Part model, mm, in its own coordinate system. A direction names the side the tool comes from. Give positions to 0.01 mm unless a question says otherwise; leave off trailing zeros. Order: outer loops, then holes, each group sorted by start corner. A loop starts at its lowest first (then second) coordinate and runs counter-clockwise, first axis right, second up. Notation, with made-up numbers: M 64.5,-13.5 L 111.5,-13.5 A25 cw 111.5,7.5 Z; hole C 21.25,51 d7. An arc over 180 degrees is marked long. One line per question, with ' | ' between items.
```python
from build123d import *

# Parameters (mm, degrees)
F0_R     = 11.4935
F0_R_2   = 9.017
F1_DEPTH = 4.064
F2_R     = 13.9954
F2_R_2   = 9.0043
F3_DEPTH = 69.85
F4_R     = 11.6713
F5_DEPTH = 7.62
F6_R     = 1.143
F7_DEPTH = 13.9964


with BuildPart() as f1:
    # F0 (on Top) → F1 (new body)
    with BuildSketch(Plane.XY):
        Circle(F0_R)
        Circle(F0_R_2, mode=Mode.SUBTRACT)
    extrude(amount=F1_DEPTH)

    # F2 (on face) → F3 (join)
    with BuildSketch(Plane(origin=(0, 0, 0), x_dir=(1, 0, 0), z_dir=(0, 0, -1))):
        Circle(F2_R)
        Circle(F2_R_2, mode=Mode.SUBTRACT)
    extrude(amount=F3_DEPTH)

    # F4 (on face) → F5 (cut)
    with BuildSketch(Plane(origin=(0, 0, -69.85), x_dir=(1, 0, 0), z_dir=(0, 0, -1))):
        Circle(F4_R)
    extrude(amount=-F5_DEPTH, mode=Mode.SUBTRACT)

    # F6 (on Right) → F7 (cut, through all)
    with BuildSketch(Plane.YZ):
        with Locations((0, -67.31)):
            Circle(F6_R)
    extrude(amount=F7_DEPTH, mode=Mode.SUBTRACT)


solid = f1.part
```
1. Slice it at D-D on z = -41. Give the cut face in (x, y).
Worked out:
outline: C 0,0 d27.99; hole C 0,0 d18.01
2. Tool access for faces 5 (the flat face through (-7, -6, 4.064)), 6 (the cylindrical face through (12.789, -0.149, -66.177)), 7 (the cylindrical face through (11.13, -3.51, -66.09)): list every direction of +Z, -Z, +X, -X, +Y, -Y with a clear straight run to the whole face (end or side of a thin tool).
Worked out:
face 5: +Z, +X, -X, +Y, -Y | face 6: +X | face 7: -Z
3. Mould opens along X. For faces 1 (the flat face through (6, 7, -62.23)), 2 (the cylindrical face through (-1.95, 8.79, -30.68)), 3 (the flat face through (2, -11.5, 0)), 4 (the cylindrical face through (6.18, 9.69, 2)) say: released by +X, released by -X, zero draft, split by the parting line, or undercut.
Worked out:
face 1: undercut | face 2: undercut | face 3: zero draft | face 4: split by the parting line
4. Drop flat-ended pins along their axis: pin 1 (1.5 mm diameter, centred on x = 8, z = -5, fed in from -Y); pin 2 (3 mm diameter, centred on y = -4.5, z = -43.5, fed in from +X); pin 3 (2 mm diameter, centred on y = 6, z = -34.5, fed in from -X). Give the stop position or say it passes through.
Worked out:
pin 1: stops at y = -11.97 | pin 2: stops at x = 13.67 | pin 3: stops at x = -13.07
5. Slice it at B-B on y = 0. Give the number of separate pieces and of enclosed holes in the cut face, then the cut area to 3 significant figures.
Worked out:
separate pieces: 3 | enclosed holes: 0 | area: 671 mm2
6. Probe L1, parallel to X at y = 0, z = -45; L2, parallel to Z at x = 12.75, y = 0. List the from-to ranges inside material, lowest first. Write a range as from..to.
Worked out:
L1: x = -14..-9, 9..14 | L2: z = -69.85..-68.45, -66.17..0
